```python
from build123d import *

# Parameters (mm, degrees)
BOSS_EXTRUDE2_DEPTH     = 120
CUT_EXTRUDE1_DEPTH      = 12.8
CUT_EXTRUDE1_DEPTH_BACK = 12.8
SKETCH5_W               = 23.4
SKETCH5_H               = 29


with BuildPart() as part:
    # Sketch4 → Boss-Extrude2 (new body)
    with BuildSketch(Plane.XY):
        with BuildLine():
            Line((-15, -15), (15, -15))
            ThreePointArc((15, -15), (17.828427125, -13.828427125), (19, -11))
            Line((19, -11), (19, 11))
            ThreePointArc((19, 11), (17.828427125, 13.828427125), (15, 15))
            Line((15, 15), (-15, 15))
            ThreePointArc((-15, 15), (-17.828427125, 13.828427125), (-19, 11))
            Line((-19, 11), (-19, -11))
            ThreePointArc((-19, -11), (-17.828427125, -13.828427125), (-15, -15))
        make_face()
    extrude(amount=BOSS_EXTRUDE2_DEPTH)

    # Sketch5 → Cut-Extrude1 (cut, two sides: drawn at the far end of the back side and taken through both)
    with BuildSketch(Plane(origin=(0, 0, 0), x_dir=(0, 0, -1), z_dir=(1, 0, 0)).offset(-CUT_EXTRUDE1_DEPTH_BACK)):
        with Locations((-60, 9.5)):
            Rectangle(SKETCH5_W, SKETCH5_H)
    extrude(amount=CUT_EXTRUDE1_DEPTH + CUT_EXTRUDE1_DEPTH_BACK, mode=Mode.SUBTRACT)


solid = part.part
```
Geometry check sheet. Reference: the model listing, model coordinates, mm. A direction names the side the tool comes from. Coordinates: 2 decimals unless noted, no trailing zeros. Write each loop counter-clockwise with the first axis right and the second up, starting at its lowest first coordinate (ties: lowest second). Pieces come first, ordered by that corner, then holes. Notation, with made-up numbers: M -23,-24.75 L 14,-24.75 A16 cw 14,-10.75 Z; hole C -9.75,22.25 d11. An arc over 180 degrees is marked long. One line per item, written item: value. Start each with the question number.
(1) Sectioned sample at C-C, the plane x = 1. Enter the section's corners in (y, z).
(2) Tool access check on faces 1 (the face through (-12.8, 5, 60)), 2 (the face through (0, 0, 0)). Record the directions out of +Z, -Z, +X, -X, +Y, -Y that give a thin tool (end or side, any length) a straight path to the whole face; none if there is none.
(3) Scan lines: line 1 along Z through (x, y) = (1, -1.25); line 2 along X through (y, z) = (3.5, 58.5); line 3 along Y through (x, z) = (3, 53). Record each from-to range of solid material in increasing order. Write a range as [from, to].
(4) Sectioned sample at B-B, the plane z = 53.5. Enter the section's corners in (x, y).
(5) Sectioned sample at A-A, the plane y = -3. Enter the section's corners in (x, z), and give its area (3 significant figures).
(6) Release check for a two-part mould opening along X. For faces 3 (the face through (0, 5, 71.7)), 4 (the face through (-19, 0, 59)), 5 (the face through (0, 15, 72)) record: released by +X, released by -X, zero draft, split by the parting line, or undercut.
Filled sheet:
1. outline: M -15,0 L 15,0 L 15,48.3 L -5,48.3 L -5,71.7 L 15,71.7 L 15,120 L -15,120 Z
2. face 1: +Y
2. face 2: -Z, +X, -X, +Y, -Y
3. line 1: [0, 48.3], [71.7, 120]
3. line 2: [-19, -12.8], [12.8, 19]
3. line 3: [-15, -5]
4. outline: M -19,-11 A4 ccw -15,-15 L 15,-15 A4 ccw 19,-11 L 19,11 A4 ccw 15,15 L 12.8,15 L 12.8,-5 L -12.8,-5 L -12.8,15 L -15,15 A4 ccw -19,11 Z
5. outline: M -19,0 L 19,0 L 19,120 L -19,120 Z; hole M -12.8,48.3 L 12.8,48.3 L 12.8,71.7 L -12.8,71.7 Z
5. area: 3,960 mm²
6. face 3: undercut
6. face 4: released by -X
6. face 5: zero draft
